```python
from build123d import *

# Parameters (mm, degrees)
F2_SIZE2 = 3
F2_SIZE  = 3


with BuildPart() as f1:
    # F0 (on Front) → F1 (revolve)
    with BuildSketch(Plane.XZ):
        with BuildLine():
            Line((18.5, 5.15), (0, 5.15))
            Line((0, 5.15), (0, 0))
            Line((0, 0), (24, 0))
            Line((24, 0), (24, 7.5))
            Line((24, 7.5), (21, 7.5))
            Line((21, 7.5), (21, 5.15))
            ThreePointArc((21, 5.15), (20.707107, 4.442893), (20, 4.15))
            Line((20, 4.15), (19.654701, 4.15))
            ThreePointArc((19.654701, 4.15), (19.154701, 4.283975), (18.788675, 4.65))
            Line((18.788675, 4.65), (18.5, 5.15))
        make_face()
    revolve(axis=Axis((12.35421, 0, 0), (1, 0, 0)))

    # F2
    f2_edges = [f1.edges().sort_by_distance(p)[0] for p in [
        (0, 0, -5.15),
    ]]
    chamfer(f2_edges, length=F2_SIZE, length2=F2_SIZE2)


solid = f1.part
```
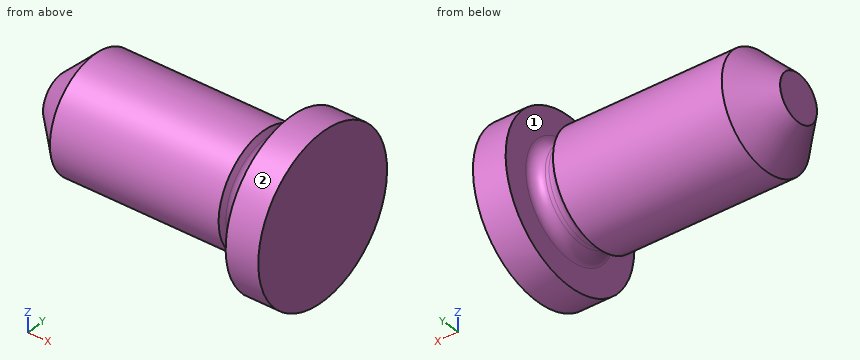
Source: CAD feature listing. Evaluate the final solid. Frame: model axes, mm. Face numbers are marked on the shaded views. A direction names the side the tool comes from. Give positions to 0.01 mm unless a question says otherwise; leave off trailing zeros. Order: outer loops, then holes, each group sorted by start corner. A loop starts at its lowest first (then second) coordinate and runs counter-clockwise, first axis right, second up.
(1) Material intervals for line 1 along Y through (x, z) = (16.5, 0.25); line 2 along Y through (x, z) = (2.5, 0); line 3 along X through (y, z) = (-1.5, 5.25), sorted ascending.
(2) Section query D-D (x = 2.5). Return the cut outline in (y, z).
(3) Contact query for flat-ended pins moving along their axis: P1, Ø8, axis at x = 16.5, z = 2.5, coming from the -Y side; P2, Ø1.5, axis at x = 5, y = -3.5, coming from the +Z side; P3, Ø3, axis at x = 12.5, y = 0.5, coming from the -Z side. Output: stop coordinate, or through.
(4) Access query for the marked faces 1 and 2. Directions: +Z, -Z, +X, -X, +Y, -Y. A direction counts if a zero-diameter tool reaches every point of the face in a straight line with its end or side. Return the directions, or none.
(5) Section query A-A (z = 0). Return the cut outline in (x, y).
(6) Section query C-C (x = 7). Return the cut outline in (y, z), plus the area to 3 significant figures.
Outcome:
1. line 1: y = -5.14 to 5.14
1. line 2: y = -4.65 to 4.65
1. line 3: x = 21 to 24
2. outline: circle Ø9.3 at (0, 0)
3. P1: stops at y = -5.15
3. P2: stops at z = 4.35
3. P3: stops at z = -5.15
4. face 1: -X
4. face 2: +X, -X
5. outline: (0, -2.15) - (3, -5.15) - (18.5, -5.15) - (18.79, -4.65) arc R1 cw to (19.65, -4.15) - (20, -4.15) arc R1 cw to (21, -5.15) - (21, -7.5) - (24, -7.5) - (24, 7.5) - (21, 7.5) - (21, 5.15) arc R1 cw to (20, 4.15) - (19.65, 4.15) arc R1 cw to (18.79, 4.65) - (18.5, 5.15) - (3, 5.15) - (0, 2.15) - close
6. outline: circle Ø10.3 at (0, 0)
6. area: 83.3 mm2
